For this review, use the dimensioned drawing (mm, ordinates from the lowest corner) and the shaded views. Round coordinates to 2 decimals unless told otherwise and drop trailing zeros. Order: outer loops, then holes, each group sorted by start corner. A loop starts at its lowest first (then second) coordinate and runs counter-clockwise, first axis right, second up. Notation, with made-up numbers: (61, 22) - (87, 22) arc R26 ccw to (87, 57) - close; hole circle Ø11 at (27, 2.25). An arc over 180 degrees is marked (long way). Write each question's results on one line, items separated by ' | '. Start each with the question number.
(1) For L1, parallel to X at y = 5.25, z = 5; L2, parallel to X at y = 6.5, z = 8; L3, parallel to Y at x = 121.92, z = 4, list the stretches that pass through material, from the lowest coordinate up. Write a range as from..to.
(2) Insertion check: pin 1 Ø4.5 at (x, y) = (5.08, 5.08) entering from +Z. The pin has a flat end and moves straight along its axis. Give the tip position at first contact, or say it passes through.
(3) Take a section at A-A, the plane z = 2.5. Give the number of separate pieces and of enclosed holes in the cut face, plus the area to 3 significant figures.
(4) Take a section at B-B, the plane y = 1.5. Give the boundary of the cut face in (x, z), plus the area to 3 significant figures.
(5) Draft analysis for pull direction Y (two halves, no side actions). For the marked faces 1, 2 and 3, state which applies: pulls with the +Y half, pulls with the -Y half, needs draft (parallel to the pull), parting line crosses it, or undercut.
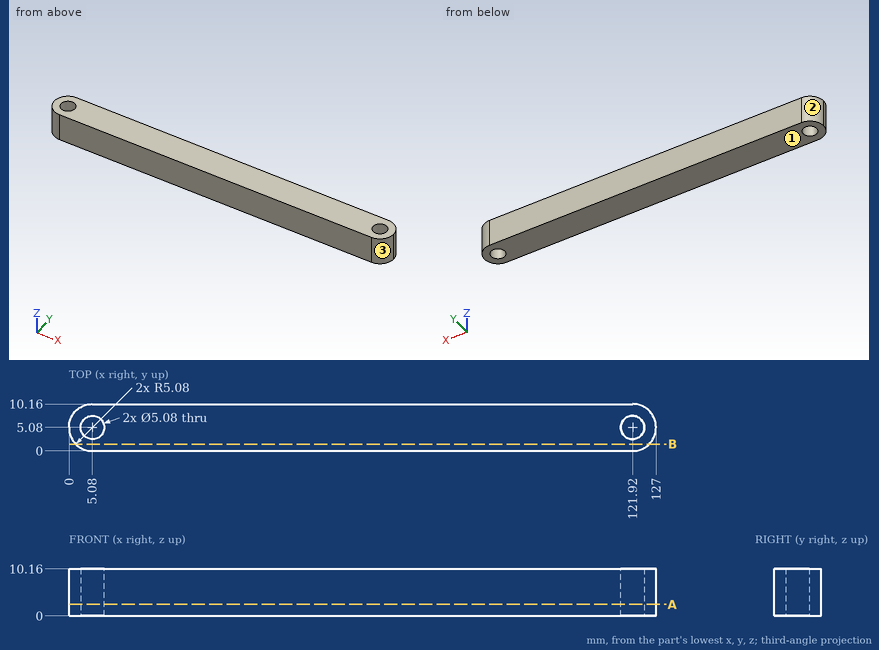
Results below:
1) L1: x = 0..2.55, 7.61..119.39, 124.45..127 | L2: x = 0.2..2.97, 7.19..119.81, 124.03..126.8 | L3: y = 0..2.54, 7.62..10.16
2) pin 1: passes through
3) separate pieces: 1 | enclosed holes: 2 | area: 1,230 mm^2
4) outline: (1.48, 0) - (125.52, 0) - (125.52, 10.16) - (1.48, 10.16) - close | area: 1,260 mm^2
5) face 1: needs draft | face 2: pulls with the +Y half | face 3: pulls with the -Y half
